```python
from build123d import *

# Parameters (mm, degrees)
ESQUISSE3_R      = 2
ESQUISSE3_R_2    = 10
EXTRUSION2_DEPTH = 19
EXTRUSION4_DEPTH = 27


with BuildPart() as part:
    # Esquisse1 → Révolution1 (revolve)
    with BuildSketch(Plane.XY):
        Polygon((-6.5, 17), (-6.5, 41), (-8.5, 41), (-8.5, 19), (-11, 19), (-11, -3), (-10, -3), (-10, 17), align=None)
    revolve(axis=Axis((0, 0, 0), (0, 1, 0)))

    # Esquisse3 → Extrusion2 (add)
    with BuildSketch(Plane(origin=(0, 19, 0), x_dir=(1, 0, 0), z_dir=(0, 1, 0))):
        with BuildLine():
            Line((-12.449899598, -13), (-7.924146363, -13))
            Line((-7.924146363, -13), (-6.438678833, -8.918711504))
            ThreePointArc((-6.438678833, -8.918711504), (0, -11), (6.438678833, -8.918711504))
            Line((6.438678833, -8.918711504), (7.924146363, -13))
            Line((7.924146363, -13), (12.449899598, -13))
            ThreePointArc((12.449899598, -13), (12.727922061, -12.727922061), (13, -12.449899598))
            Line((13, -12.449899598), (13, -7.924146363))
            Line((13, -7.924146363), (8.918711504, -6.438678833))
            ThreePointArc((8.918711504, -6.438678833), (11, 0), (8.918711504, 6.438678833))
            Line((8.918711504, 6.438678833), (13, 7.924146363))
            Line((13, 7.924146363), (13, 12.449899598))
            ThreePointArc((13, 12.449899598), (12.727922061, 12.727922061), (12.449899598, 13))
            Line((12.449899598, 13), (7.924146363, 13))
            Line((7.924146363, 13), (6.438678833, 8.918711504))
            ThreePointArc((6.438678833, 8.918711504), (0, 11), (-6.438678833, 8.918711504))
            Line((-6.438678833, 8.918711504), (-7.924146363, 13))
            Line((-7.924146363, 13), (-12.449899598, 13))
            ThreePointArc((-12.449899598, 13), (-12.727922061, 12.727922061), (-13, 12.449899598))
            Line((-13, 12.449899598), (-13, 7.924146363))
            Line((-13, 7.924146363), (-8.918711504, 6.438678833))
            ThreePointArc((-8.918711504, 6.438678833), (-11, 0), (-8.918711504, -6.438678833))
            Line((-8.918711504, -6.438678833), (-13, -7.924146363))
            Line((-13, -7.924146363), (-13, -12.449899598))
            ThreePointArc((-13, -12.449899598), (-12.727922061, -12.727922061), (-12.449899598, -13))
        make_face()
        with Locations((10.606601718, 10.606601718)):
            Circle(ESQUISSE3_R, mode=Mode.SUBTRACT)
        with Locations((-10.606601718, -10.606601718)):
            Circle(ESQUISSE3_R, mode=Mode.SUBTRACT)
        with Locations((-10.606601718, 10.606601718)):
            Circle(ESQUISSE3_R, mode=Mode.SUBTRACT)
        with Locations((10.606601718, -10.606601718)):
            Circle(ESQUISSE3_R, mode=Mode.SUBTRACT)
        Circle(ESQUISSE3_R_2, mode=Mode.SUBTRACT)
    extrude(amount=-EXTRUSION2_DEPTH)

    # Esquisse4 → Extrusion4 (cut, through all)
    with BuildSketch(Plane.XY.offset(13)):
        with BuildLine():
            Line((-1, 37), (-1, 12))
            ThreePointArc((-1, 12), (0, 11), (1, 12))
            Line((1, 12), (1, 37))
            ThreePointArc((1, 37), (0, 38), (-1, 37))
        make_face()
    extrude(amount=-EXTRUSION4_DEPTH, mode=Mode.SUBTRACT)


solid = part.part
```
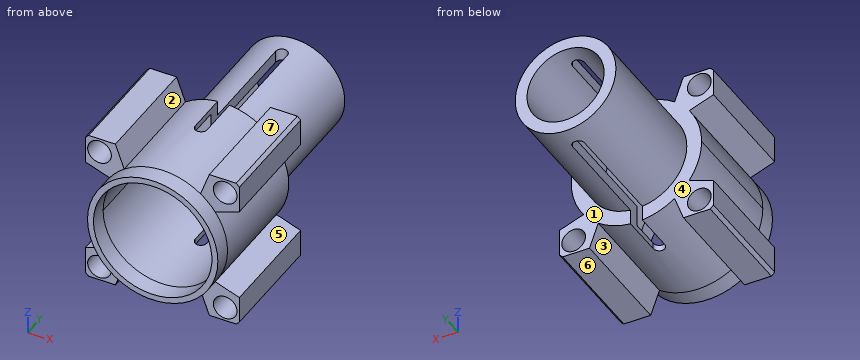
Geometry: final body of the model. Coordinates: model frame, mm. Face numbers are marked on the shaded views. A direction names the side the tool comes from. Coordinates: 2 decimals unless noted, no trailing zeros. Order: outer loops, then holes, each group sorted by start corner. A loop starts at its lowest first (then second) coordinate and runs counter-clockwise, first axis right, second up. Notation, with made-up numbers: (40.5, -19) -> (74.5, -19) arc R20 cw to (74.5, 11) -> close; hole circle Ø9 at (-8.5, 52). An arc over 180 degrees is marked (long way). Write item = value, one per line.
(1) Pull-direction query (Z, two-part tool) for the marked faces 5, 6 and 7; classes: pulls with the +Z half, pulls with the -Z half, needs draft (parallel to the pull), parting line crosses it, or undercut.
Solved:
face_5 = undercut
face_6 = pulls with the -Z half
face_7 = pulls with the +Z half
(2) Cut plane B-B on x = 4.75. Return loops of the section in (y, z).
Solved:
outline = (-3, -9.92) -> (19, -9.92) -> (19, -7.05) -> (41, -7.05) -> (41, -4.44) -> (17, -4.44) -> (17, -8.8) -> (-3, -8.8) -> close; (-3, 8.8) -> (17, 8.8) -> (17, 4.44) -> (41, 4.44) -> (41, 7.05) -> (19, 7.05) -> (19, 9.92) -> (-3, 9.92) -> close
(3) Cut plane D-D on y = 29. Return loops of the section in (x, z).
Solved:
outline = (-1, -8.44) -> (-1, -6.42) arc R6.5 cw to (-1, 6.42) -> (-1, 8.44) arc R8.5 ccw to start; (1, -8.44) arc R8.5 ccw to (1, 8.44) -> (1, 6.42) arc R6.5 cw to (1, -6.42) -> close
(4) Cut plane A-A on x = 0. Return loops of the section in (y, z), plus the area to 3 significant figures.
Solved:
outline = (-3, -11) -> (11, -11) -> (11, -10) -> (-3, -10) -> close; (-3, 10) -> (11, 10) -> (11, 11) -> (-3, 11) -> close; (38, -8.5) -> (41, -8.5) -> (41, -6.5) -> (38, -6.5) -> close; (38, 6.5) -> (41, 6.5) -> (41, 8.5) -> (38, 8.5) -> close
area = 40.0 mm²
(5) Cut plane C-C on z = -1.25. Return loops of the section in (x, y).
Solved:
outline = (-10.93, -3) -> (-9.92, -3) -> (-9.92, 17) -> (-6.38, 17) -> (-6.38, 41) -> (-8.41, 41) -> (-8.41, 19) -> (-10.93, 19) -> close; (6.38, 17) -> (9.92, 17) -> (9.92, -3) -> (10.93, -3) -> (10.93, 19) -> (8.41, 19) -> (8.41, 41) -> (6.38, 41) -> close
(6) Line query: line 1 (X direction, y = 31.5, z = 0); line 2 (X direction, y = -1.85, z = 0); line 3 (Y direction, x = 5.25, z = 6.75). Output: solid intervals per line, ascending.
Solved:
line_1 = -8.5 to -6.5, 6.5 to 8.5
line_2 = -11 to -10, 10 to 11
line_3 = 17 to 19
(7) Pin query (flat end, axial travel): pin 1 Ø12 at (y, z) = (29.5, -10) entering from -X; pin 2 Ø8 at (y, z) = (29.5, 9) entering from -X; pin 3 Ø3.5 at (x, z) = (-8.5, -10) entering from -Y; pin 4 Ø12 at (x, y) = (2.5, 6) entering from +Z. Return the tip coordinate at first contact, or that it passes through.
Solved:
pin_1 = -7.5
pin_2 = -6.87
pin_3 = 0
pin_4 = 13
(8) Access query for the marked faces 1, 2, 3 and 4. Directions: +Z, -Z, +X, -X, +Y, -Y. A direction counts if a zero-diameter tool reaches every point of the face in a straight line with its end or side. Return the directions, or none.
Solved:
face_1 = +X, +Y
face_2 = +Z, +Y, -Y
face_3 = -Z, +Y, -Y
face_4 = -X, +Y
